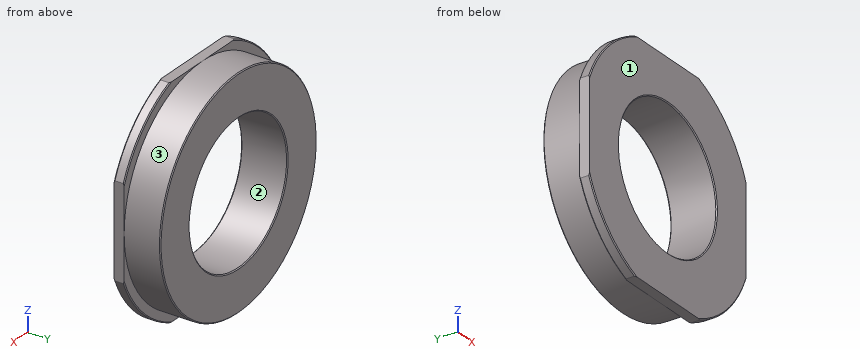
```python
from build123d import *

# Parameters (mm, degrees)
SKETCH_1_R          = 13
EXTRUDE_1_DEPTH     = 1.1
SKETCH_2_R          = 12
EXTRUDE_2_DEPTH     = 3.9
SKETCH_3_R          = 7.5
CUT_EXTRUDE_1_DEPTH = 20.052558883
CHAMFER_1_SIZE      = 0.1
CUT_EXTRUDE_2_DEPTH = 19.793881983


with BuildPart() as part:
    # 草图1 → 凸台-拉伸1 (new body)
    with BuildSketch(Plane(origin=(0, 0, 0), x_dir=(1, 0, 0), z_dir=(0, 1, 0))):
        with Locations(Location((0, 0, 0), (0, 0, 270))):
            Circle(SKETCH_1_R)
    extrude(amount=EXTRUDE_1_DEPTH)

    # 草图2 → 凸台-拉伸2 (add)
    with BuildSketch(Plane(origin=(0, 1.1, 0), x_dir=(1, 0, 0), z_dir=(0, 1, 0))):
        with Locations(Location((0, 0, 0), (0, 0, 270))):
            Circle(SKETCH_2_R)
    extrude(amount=EXTRUDE_2_DEPTH)

    # 草图3 → 切除-拉伸1 (cut, through all)
    with BuildSketch(Plane(origin=(0, 5, 0), x_dir=(1, 0, 0), z_dir=(0, 1, 0))):
        with Locations(Location((0, 0, 0), (0, 0, 270))):
            Circle(SKETCH_3_R)
    extrude(amount=-CUT_EXTRUDE_1_DEPTH, mode=Mode.SUBTRACT)

    # 倒角1
    chamfer_1_edges = [part.edges().sort_by_distance(p)[0] for p in [
        (0, 0, -7.5),
        (0, 5, -7.5),
        (0, 0, -13),
        (0, 1.1, -13),
        (0, 5, -12),
    ]]
    chamfer(chamfer_1_edges, length=CHAMFER_1_SIZE)

    # 草图7 → 切除-拉伸2 (cut, through all)
    with BuildSketch(Plane(origin=(0, 1.1, 0), x_dir=(1, 0, 0), z_dir=(0, 1, 0))):
        with BuildLine():
            Line((-5, 12), (5, 12))
            ThreePointArc((5, 12), (0, 13), (-5, 12))
        make_face()
        with BuildLine():
            Line((-12, 5), (-12, -5))
            ThreePointArc((-12, -5), (-13, 0), (-12, 5))
        make_face()
        with BuildLine():
            Line((-5, -12), (5, -12))
            ThreePointArc((5, -12), (0, -13), (-5, -12))
        make_face()
        with BuildLine():
            Line((12, 5), (12, -5))
            ThreePointArc((12, -5), (13, 0), (12, 5))
        make_face()
    extrude(amount=-CUT_EXTRUDE_2_DEPTH, mode=Mode.SUBTRACT)


solid = part.part
```
Here's how the part is built. I have some questions about the finished solid (model axes, mm). Face numbers are marked on the shaded views. Round coordinates to 2 decimals unless told otherwise and drop trailing zeros. Write each loop counter-clockwise with the first axis right and the second up, starting at its lowest first coordinate (ties: lowest second). Pieces come first, ordered by that corner, then holes. Notation, with made-up numbers: M 32.25,56 L 74.25,56 A23 ccw 74.25,64 Z; hole C 64,46 d2. An arc over 180 degrees is marked long. Answer as CSV lines item,"result". Start each with the question number.
1. Suppose I cut it at A-A on y = 2.6. Write out the boundary of the cut face in (x, z).
2. I need wall thicknesses on probe 1 along X at (y, z) = (1.8, 0); probe 2 along Z at (x, y) = (4.5, 4.8); probe 3 along X at (y, z) = (3.65, 2.5). Which ranges of each line are inside material? Lowest first, please.
3. Thinking about a two-plate mould opening in X: for the marked faces 1, 2 and 3, which applies, released by +X, released by -X, zero draft, split by the parting line, or undercut?
4. I'm going to push flat-ended pins straight in: pin 1 Ø2 at (y, z) = (4, 5) entering from -X; pin 2 Ø3 at (y, z) = (4, 2) entering from +X; pin 3 Ø1 at (x, y) = (-6, 1) entering from +Z. Where does each tip first touch, or does it pass through?
Check result:
1,outline,"C 0,0 d24; hole C 0,0 d15"
2,probe 1,"x = -12 to -7.5, 7.5 to 12"
2,probe 2,"z = -11.12 to -6, 6 to 11.12"
2,probe 3,"x = -11.74 to -7.07, 7.07 to 11.74"
3,face 1,"zero draft"
3,face 2,"undercut"
3,face 3,"split by the parting line"
4,pin 1,"stops at x = -11.31"
4,pin 2,"stops at x = 11.99"
4,pin 3,"stops at z = 11.78"
